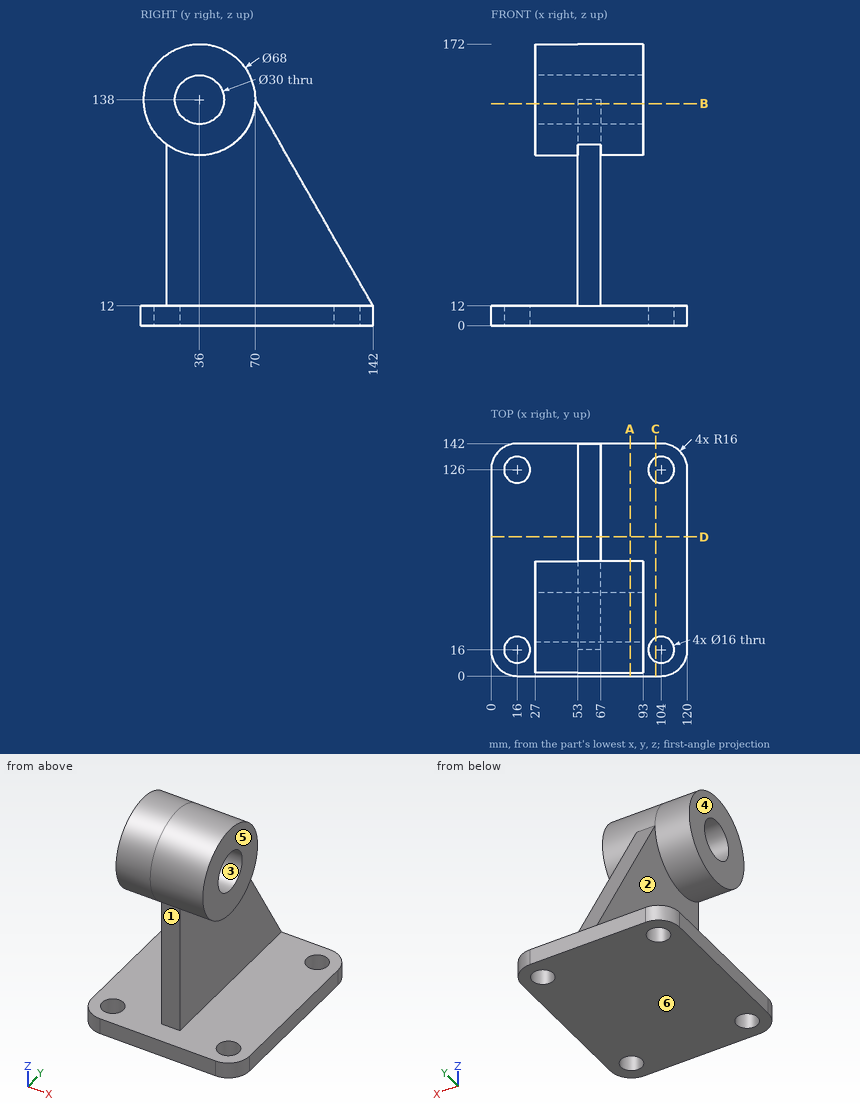
Study the drawing (mm; zero at the part's minimum x, y, z) and answer. A direction names the side the tool comes from. Coordinates: 2 decimals unless noted, no trailing zeros. Write each loop counter-clockwise with the first axis right and the second up, starting at its lowest first coordinate (ties: lowest second). Pieces come first, ordered by that corner, then holes. Notation, with made-up numbers: (52, -21.5) -> (76, -21.5) arc R12 ccw to (76, 1.5) -> close; hole circle Ø6 at (14, 80). An arc over 180 degrees is marked (long way). Write each question's results on one line, items separated by ' | '. Start each with the question number.
1) For a pull along Y with two mould halves and no side action, classify the marked faces 1, 2 and 3 as +Y half, -Y half, draft (parallel to the pull), parting line (faces both ways), or undercut.
2) Straight lines are drawn through the part: probe 1 along Z at (x, y) = (74.5, 36); probe 2 along Z at (x, y) = (81, 25); probe 3 along X at (y, z) = (65.5, 107.5). For each, find the intervals that lie inside material, in ascending order.
3) Flat-ended cylindrical pins translate along their axes: pin 1 Ø10 at (y, z) = (103, 42.5) entering from -X; pin 2 Ø4 at (x, y) = (89, 72.5) entering from +Z; pin 3 Ø1 at (x, z) = (56, 112.5) entering from -Y. Find the tip coordinate at first contact, or state that the pin passes through.
4) A tool of negligible diameter and unlimited length cuts with its end or side. For the marked faces 4, 5 and 6, from which of +Z, -Z, +X, -X, +Y, -Y can it reach the whole face along a straight path? Write none if from no direction.
5) A cutting plane is placed at D-D (y = 85). Determine the outline of the cut face in (x, z).
6) A cutting plane is placed at C-C (x = 100.5). Determine the outline of the cut face in (y, z).
7) A cutting plane is placed at A-A (x = 85). Determine the outline of the cut face in (y, z).
8) A cutting plane is placed at B-B (z = 135.5). Determine the outline of the cut face in (x, y), then the cut area to 3 significant figures.
Values follow:
1) face 1: -Y half | face 2: draft | face 3: undercut
2) probe 1: 0 to 12, 104 to 123, 153 to 172 | probe 2: 0 to 12, 105.83 to 127.8, 148.2 to 170.17 | probe 3: 53 to 67
3) pin 1: x = 53 | pin 2: z = 12 | pin 3: y = 12.96
4) face 4: +Z, -X, +Y, -Y | face 5: +Z, +X, +Y, -Y | face 6: -Z, +X, -X, +Y, -Y
5) outline: (0, 0) -> (120, 0) -> (120, 12) -> (67, 12) -> (67, 111.75) -> (53, 111.75) -> (53, 12) -> (0, 12) -> close
6) outline: (0, 0) -> (8.81, 0) -> (8.81, 12) -> (0, 12) -> close; (23.19, 0) -> (118.81, 0) -> (118.81, 12) -> (23.19, 12) -> close; (133.19, 0) -> (142, 0) -> (142, 12) -> (133.19, 12) -> close
7) outline: (0, 0) -> (142, 0) -> (142, 12) -> (0, 12) -> close; circle Ø68 at (36, 138); hole circle Ø30 at (36, 138)
8) outline: (27, 2.09) -> (93, 2.09) -> (93, 21.21) -> (27, 21.21) -> close; (27, 50.79) -> (93, 50.79) -> (93, 69.91) -> (67, 69.91) -> (67, 71.43) -> (53, 71.43) -> (53, 69.91) -> (27, 69.91) -> close | area: 2,540 mm²
